from build123d import *

# Parameters (mm, degrees)
RESSALTO_EXTRUS_O1_DEPTH = 100
CORTE_EXTRUS_O1_DEPTH    = 100
ESBO_O4_W                = 6
ESBO_O4_H                = 10
CORTE_EXTRUS_O3_DEPTH    = 100
ESBO_O6_W                = 4.394129168
ESBO_O6_H                = 9.553687289
ESBO_O6_W_2              = 4.232922622
ESBO_O6_H_2              = 9.401185036
ESBO_O6_H_3              = 9.804760869
CORTE_EXTRUS_O4_DEPTH    = 2
CORTE_EXTRUS_O5_DEPTH    = 9.804760869
CORTE_EXTRUS_O6_DEPTH    = 9.401185036
CORTE_EXTRUS_O7_DEPTH    = 9.553687289
RESSALTO_EXTRUS_O2_DEPTH = 2.8
RESSALTO_EXTRUS_O3_DEPTH = 2.8
CHANFRO1_SIZE            = 1
CHANFRO1_SIZE2           = 1.673157185
ESBO_O12_R               = 2
CORTE_EXTRUS_O8_DEPTH    = 5
ESBO_O14_W               = 6.5
ESBO_O14_H               = 6.5
RESSALTO_EXTRUS_O4_DEPTH = 12.5
CORTE_EXTRUS_O9_DEPTH    = 100
ESBO_O17_R               = 1.6
CORTE_EXTRUS_O10_DEPTH   = 100
FILETE1_R                = 1
ESBO_O18_W               = 5
ESBO_O18_H               = 4
CORTE_EXTRUS_O11_DEPTH   = 5
CHANFRO2_SIZE            = 5


with BuildPart() as part:
    # Esboço1 → Ressalto-extrusão1 (new body)
    with BuildSketch(Plane.XY):
        Polygon((51, -6.786066874), (51, -20.786066874), (26.272703225, -11.786066874), (26.272703225, -6.786066874), align=None)
    extrude(amount=-RESSALTO_EXTRUS_O1_DEPTH)

    # Esboço2 → Corte-extrusão1 (cut)
    with BuildSketch(Plane.XY):
        Polygon((34.3, -12.026146103), (26.272703225, -9.786066874), (26.272703225, -6.786066874), (51, -6.786066874), (51, -12.026146103), (49.5, -12.026146103), align=None)
    extrude(amount=-CORTE_EXTRUS_O1_DEPTH, mode=Mode.SUBTRACT)

    # Esboço4 → Corte-extrusão3 (cut)
    with BuildSketch(Plane(origin=(0, -12.026146103, 0), x_dir=(1, 0, 0), z_dir=(0, 1, 0))):
        with Locations((44.8, 91.726127663)):
            Rectangle(ESBO_O4_W, ESBO_O4_H)
        with Locations((44.8, 50.226127663)):
            Rectangle(ESBO_O4_W, ESBO_O4_H)
        with Locations((44.8, 8.5)):
            Rectangle(ESBO_O4_W, ESBO_O4_H)
    extrude(amount=-CORTE_EXTRUS_O3_DEPTH, mode=Mode.SUBTRACT)

    # Esboço6 → Corte-extrusão4 (cut)
    with BuildSketch(Plane(origin=(0, -12.026146103, 0), x_dir=(1, 0, 0), z_dir=(0, 1, 0))):
        with Locations((36.946648007, 91.760642218)):
            Rectangle(ESBO_O6_W, ESBO_O6_H)
        with Locations((37.02725128, 50.165247763)):
            Rectangle(ESBO_O6_W_2, ESBO_O6_H_2)
        with Locations((37.02725128, 8.595463062)):
            Rectangle(ESBO_O6_W_2, ESBO_O6_H_3)
    extrude(amount=-CORTE_EXTRUS_O4_DEPTH, mode=Mode.SUBTRACT)

    # Esboço7 → Corte-extrusão5 (cut)
    with BuildSketch(Plane.XY.offset(-13.497843496)):
        Polygon((34.910789969, -12.026146103), (34.910789969, -14.026146103), (31.643973079, -11.284961255), align=None)
    extrude(amount=CORTE_EXTRUS_O5_DEPTH, mode=Mode.SUBTRACT)

    # Esboço8 → Corte-extrusão6 (cut)
    with BuildSketch(Plane.XY.offset(-54.865840281)):
        Polygon((34.910789969, -14.026146103), (34.910789969, -12.026146103), (31.335529191, -11.026146103), align=None)
    extrude(amount=CORTE_EXTRUS_O6_DEPTH, mode=Mode.SUBTRACT)

    # Esboço9 → Corte-extrusão7 (cut)
    with BuildSketch(Plane.XY.offset(-96.537485862)):
        Polygon((34.749583423, -14.026146103), (34.749583423, -12.026146103), (30.165579372, -10.179709995), align=None)
    extrude(amount=CORTE_EXTRUS_O7_DEPTH, mode=Mode.SUBTRACT)

    # Esboço10 → Ressalto-extrusão2 (add)
    with BuildSketch(Plane.XY):
        Polygon((51, -12.026146103), (51, 9.973853897), (51, 12.713933126), (49.541118417, 12.747281328), (45.801947659, 12.747281328), (33, 15.973853897), (34.3, -12.026146103), align=None)
    extrude(amount=-RESSALTO_EXTRUS_O2_DEPTH)

    # Esboço11 → Ressalto-extrusão3 (add)
    with BuildSketch(Plane(origin=(0, 0, -100), x_dir=(-1, 0, 0), z_dir=(0, 0, -1))):
        Polygon((-34.3, -12.026146103), (-33, 15.973853897), (-45.271603303, 12.747281328), (-49.541118417, 12.747281328), (-51, 12.713933126), (-51, -12.026146103), align=None)
    extrude(amount=-RESSALTO_EXTRUS_O3_DEPTH)

    # Chanfro1
    chanfro1_edges = [part.edges().sort_by_distance(p)[0] for p in [
        (26.272703225, -11.786066874, -50),
    ]]
    chanfro1_side = [part.faces().sort_by_distance(p)[0] for p in [
        (38.152449511, -16.109940913, -49.988164623),
    ]]
    chamfer(chanfro1_edges, length=CHANFRO1_SIZE, length2=CHANFRO1_SIZE2, reference=chanfro1_side[0])

    # Esboço12 → Corte-extrusão8 (cut)
    with BuildSketch(Plane(origin=(51, 0, 0), x_dir=(0, 0, -1), z_dir=(1, 0, 0))):
        with Locations((75, -15.026146103)):
            Circle(ESBO_O12_R)
        with Locations((25, -15.026146103)):
            Circle(ESBO_O12_R)
    extrude(amount=-CORTE_EXTRUS_O8_DEPTH, mode=Mode.SUBTRACT)

    # Esboço14 → Ressalto-extrusão4 (add)
    with BuildSketch(Plane(origin=(51, 0, 0), x_dir=(0, 0, -1), z_dir=(1, 0, 0))):
        with Locations((6.05, 9.463933126)):
            Rectangle(ESBO_O14_W, ESBO_O14_H)
        with Locations((93.95, 9.463933126)):
            Rectangle(ESBO_O14_W, ESBO_O14_H)
    extrude(amount=-RESSALTO_EXTRUS_O4_DEPTH)

    # Esboço15 → Corte-extrusão9 (cut)
    with BuildSketch(Plane.XY):
        with BuildLine():
            ThreePointArc((33, 15.973853897), (41.611155482, 12.19684706), (51, 12.713933126))
            ThreePointArc((51, 12.713933126), (42.289458716, 15.942170666), (33, 15.973853897))
        make_face()
    extrude(amount=-CORTE_EXTRUS_O9_DEPTH, mode=Mode.SUBTRACT)

    # Esboço17 → Corte-extrusão10 (cut)
    with BuildSketch(Plane.ZY.offset(-38.5)):
        with Locations((-6.05, 9.213933126)):
            Circle(ESBO_O17_R)
        with Locations((-93.95, 9.213933126)):
            Circle(ESBO_O17_R)
    extrude(amount=-CORTE_EXTRUS_O10_DEPTH, mode=Mode.SUBTRACT)

    # Filete1
    filete1_edges = [part.edges().sort_by_distance(p)[0] for p in [
        (44.75, 6.213933126, -2.8),
        (44.75, 6.213933126, -9.3),
        (44.75, 6.213933126, -97.2),
        (44.75, 6.213933126, -90.7),
    ]]
    fillet(filete1_edges, radius=FILETE1_R)

    # Esboço18 → Corte-extrusão11 (cut)
    with BuildSketch(Plane(origin=(0, -12.026146103, 0), x_dir=(1, 0, 0), z_dir=(0, 1, 0))):
        with Locations((48.5, 17)):
            Rectangle(ESBO_O18_W, ESBO_O18_H)
        with Locations((48.5, 83)):
            Rectangle(ESBO_O18_W, ESBO_O18_H)
    extrude(amount=-CORTE_EXTRUS_O11_DEPTH, mode=Mode.SUBTRACT)

    # Chanfro2
    chanfro2_edges = [part.edges().sort_by_distance(p)[0] for p in [
        (46, -17.026146103, -83),
        (46, -17.026146103, -17),
    ]]
    chamfer(chanfro2_edges, length=CHANFRO2_SIZE - 0.0001)  # a hair under: the kernel refuses the full size


solid = part.part
The listing builds one solid part. Answer for the finished solid, in the listing's coordinates (mm). A direction names the side the tool comes from. Give positions to 0.01 mm unless a question says otherwise; leave off trailing zeros. Order: outer loops, then holes, each group sorted by start corner. A loop starts at its lowest first (then second) coordinate and runs counter-clockwise, first axis right, second up. Notation, with made-up numbers: (31, -3) -> (81, -3) arc R37 cw to (81, 36) -> close; hole circle Ø11 at (68, 54). An arc over 180 degrees is marked (long way). Put each result on its own line as item: value.
Item 1: For faces 3 (the face through (36, -13, -54.866)), 4 (the face through (45, -15, -96.726)), 5 (the face through (36, -13, -96.537)), 6 (the face through (49, -14, -15)), 7 (the face through (46, -15, -75)), determine the directions among +Z, -Z, +X, -X, +Y, -Y from which every point of the face is accessible in a straight line to the end or side of a thin tool.
Established:
face 3: +Y
face 4: -Y
face 5: none
face 6: +X, +Y
face 7: +X
Item 2: A cutting plane is placed at A-A on z = -6.05. Give the vertices of the cut face in (x, y), plus the area to 3 significant figures.
Established:
outline: (26.27, -10.11) -> (27.21, -12.13) -> (41.8, -17.44) -> (41.8, -12.03) -> (39.14, -12.03) -> (39.14, -14.03) -> (34.91, -14.03) -> (31.64, -11.28) -> (26.27, -9.79) -> close; (38.5, 6.21) -> (51, 6.21) -> (51, 7.61) -> (38.5, 7.61) -> close; (38.5, 10.81) -> (51, 10.81) -> (51, 12.71) arc R20.26 cw to (39.44, 12.71) -> (38.5, 12.71) -> close; (47.8, -19.62) -> (51, -20.79) -> (51, -12.03) -> (47.8, -12.03) -> close
area: 97.8 mm^2
Item 3: A cutting plane is placed at D-D on z = -25. Give the vertices of the cut face in (x, y).
Established:
outline: (26.27, -10.11) -> (27.21, -12.13) -> (51, -20.79) -> (51, -17.03) -> (46, -17.03) -> (46, -13.03) -> (51, -13.03) -> (51, -12.03) -> (34.3, -12.03) -> (26.27, -9.79) -> close
Item 4: Straight lines are drawn through the part: line 1 (Z direction, x = 33.75, y = -13); line 2 (Z direction, x = 46, y = -1); line 3 (Y direction, x = 49.9, z = -25). For each, find the intervals that lie inside material, in ascending order.
Established:
line 1: z = -100 to -96.54, -86.98 to -54.87, -45.46 to -13.5, -3.69 to 0
line 2: z = -100 to -97.2, -2.8 to 0
line 3: y = -20.39 to -17.03, -13.03 to -12.03
Item 5: Given P1, Ø1.2, axis at y = -16, z = -25.5, coming from the +X side; P2, Ø12, axis at x = 42.5, z = -59.5, coming from the +Y side; P3, Ø1.4, axis at x = 43.5, z = -6, coming from the -Y side; P4, Ø10, axis at y = -4, z = -82, coming from the -X side, each flat-ended and moving along its own axis, determine where each tip first touches the part or whether it passes through.
Established:
P1: stops at x = 46
P2: stops at y = -12.03
P3: stops at y = 6.21
P4: passes through
Item 6: A cutting plane is placed at B-B on x = 44. Count the separate pieces of the cut face and the enclosed holes in it, plus the area to 3 significant figures.
Established:
separate pieces: 4
enclosed holes: 2
area: 627 mm^2
Item 7: A cutting plane is placed at C-C on y = 3.5. Give the vertices of the cut face in (x, z).
Established:
outline: (33.58, -100) -> (51, -100) -> (51, -97.2) -> (33.58, -97.2) -> close; (33.58, -2.8) -> (51, -2.8) -> (51, 0) -> (33.58, 0) -> close
Item 8: For a pull along Z with two mould halves and no side action, classify faces 1 (the face through (45, -15, -55.226)), 2 (the face through (33.66, 1.78, -98.62)) as released by +Z, released by -Z, zero draft, split by the parting line, or undercut.
Established:
face 1: undercut
face 2: zero draft
